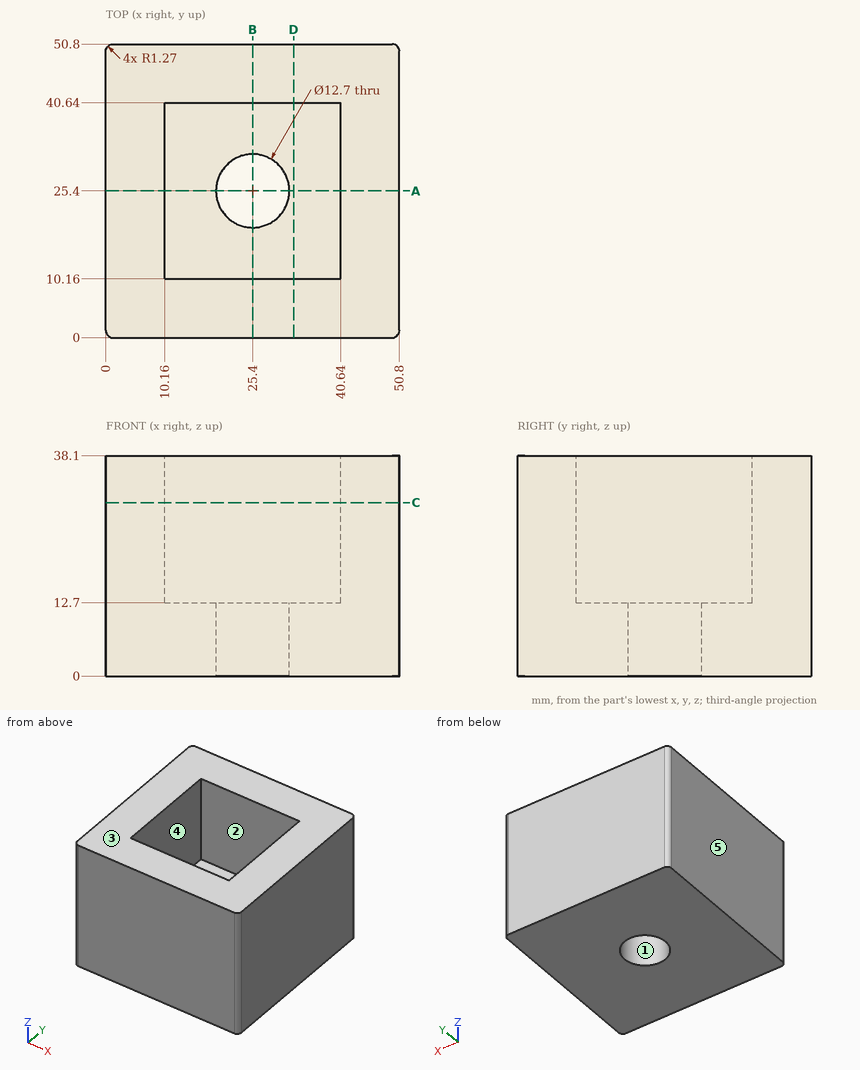
Source: three-view drawing plus pictorial views. Frame: mm from the lowest corner of the part. A direction names the side the tool comes from. Round coordinates to 2 decimals unless told otherwise and drop trailing zeros. Loops run counter-clockwise (first coordinate to the right, second up) from the corner with the lowest first, then second, coordinate; pieces in that order, holes last. Notation, with made-up numbers: M 57,-11.75 L 77,-11.75 A15 cw 77,6.25 Z; hole C -18,34 d9. An arc over 180 degrees is marked long. Answer as CSV lines item,"result".
Q1. Line query: line 1 along Y through (x, z) = (25, 6); line 2 along X through (y, z) = (33.5, 29). Output: solid intervals per line, ascending.
Verdict:
line 1,"y = 0 to 19.06, 31.74 to 50.8"
line 2,"x = 0 to 10.16, 40.64 to 50.8"
Q2. Cut plane A-A (y = 25.4). Return the cut outline in (x, z), plus the area to 4 significant figures.
Verdict:
outline,"M 0,0 L 19.05,0 L 19.05,12.7 L 10.16,12.7 L 10.16,38.1 L 0,38.1 Z; M 31.75,0 L 50.8,0 L 50.8,38.1 L 40.64,38.1 L 40.64,12.7 L 31.75,12.7 Z"
area,"1,000 mm^2"
Q3. Cut plane D-D (x = 32.5). Return the cut outline in (y, z).
Verdict:
outline,"M 0,0 L 50.8,0 L 50.8,38.1 L 40.64,38.1 L 40.64,12.7 L 10.16,12.7 L 10.16,38.1 L 0,38.1 Z"
Q4. Cut plane C-C (z = 30). Return the cut outline in (x, y), plus the area to 3 significant figures.
Verdict:
outline,"M 0,1.27 A1.27 ccw 1.27,0 L 49.53,0 A1.27 ccw 50.8,1.27 L 50.8,49.53 A1.27 ccw 49.53,50.8 L 1.27,50.8 A1.27 ccw 0,49.53 Z; hole M 10.16,10.16 L 40.64,10.16 L 40.64,40.64 L 10.16,40.64 Z"
area,"1,650 mm^2"
Q5. Reachability of the marked faces 1 and 2 from +Z, -Z, +X, -X, +Y, -Y: full face, straight path, thin tool, end or side. Return the list, or none.
Verdict:
face 1,"+Z, -Z"
face 2,"+Z"
Q6. Pull-direction query (X, two-part tool) for the marked faces 3, 4 and 5; classes: +X half, -X half, draft (parallel to the pull), parting line (faces both ways), or undercut.
Verdict:
face 3,"draft"
face 4,"undercut"
face 5,"-X half"
Q7. Contact query for a flat-ended pin moving along its axis: pin 1 (15 mm diameter, centred on x = 26, y = 27.5, fed in from +Z). Output: stop coordinate, or through.
Verdict:
pin 1,"stops at z = 12.7"
